```python
from build123d import *

# Parameters (mm, degrees)
F0_R     = 228.6
F3_DEPTH = 57.15
F4_DEPTH = 57.15


with BuildPart() as f2:
    # F2: sweep along a path in F1
    with BuildLine(Plane.XY) as f2_path:
        ThreePointArc((0, 457.2), (-323.2892203585, 323.2892203585), (-457.2, 0))
    # F0 (on Front) → F2 (sweep)
    with BuildSketch(Plane.XZ):
        with Locations((-685.8, 0)):
            Circle(F0_R)
    sweep(path=f2_path.line)

    # F3 (add): a face of the model
    f3_faces = [f2.faces().sort_by_distance(p)[0] for p in [
        (-685.8, 0, 0),
    ]]
    extrude(f3_faces, amount=F3_DEPTH)

    # F4 (add): a face of the model
    f4_faces = [f2.faces().sort_by_distance(p)[0] for p in [
        (0, 685.8, 0),
    ]]
    extrude(f4_faces, amount=F4_DEPTH)


solid = f2.part
```
Can you work these out from the model? Positions are in its coordinate system, mm. A direction names the side the tool comes from. Round coordinates to 2 decimals unless told otherwise and drop trailing zeros. Loops run counter-clockwise (first coordinate to the right, second up) from the corner with the lowest first, then second, coordinate; pieces in that order, holes last. Notation, with made-up numbers: (-27, 11) -> (18, 11) arc R23 cw to (18, 31) -> close; hole circle Ø3 at (-2, -27). An arc over 180 degrees is marked (long way). One line per item, written item: value. Start each with the question number.
1. If we section it at A-A, the plane z = 0: Write out the boundary of the cut face in (x, y), then the cut area to 3 significant figures.
2. If we section it at B-B, the plane z = -73: Write out the boundary of the cut face in (x, y).
3. If I drill on probe 1 along Y at (x, z) = (-88.5, -179); probe 2 along X at (y, z) = (804, -131); probe 3 along Y at (x, z) = (-276, -75), over which ranges is the centre line in solid material (lowest first)?
4. For faces 1 (the cylindrical face through (-854.288, -28.175, -154.499)), 2 (the flat face through (57.15, 689, 3)), 3 (the cylindrical face through (28.17, 562.91, -192.76)), which set-ups out of +Z, -Z, +X, -X, +Y, -Y let a thin tool reach every point of the face, with its end or its side?
5. For pin 1 (6 mm diameter, centred on x = -130, y = 644, fed in from -Z); pin 2 (1.5 mm diameter, centred on x = -151.5, y = 459.5, fed in from -Z); pin 3 (8 mm diameter, centred on x = -394, y = 596.5, fed in from +Z), each with a flat end and sliding along its axis, tell me the tip position at first contact or that it passes through.
Calculated:
1. outline: (-914.4, -57.15) -> (-457.2, -57.15) -> (-457.2, 0) arc R457.2 cw to (0, 457.2) -> (57.15, 457.2) -> (57.15, 914.4) -> (0, 914.4) arc R914.4 ccw to (-914.4, 0) -> close
1. area: 545,000 mm²
2. outline: (-902.43, -57.15) -> (-469.17, -57.15) -> (-469.17, 0) arc R469.17 cw to (0, 469.17) -> (57.15, 469.17) -> (57.15, 902.43) -> (0, 902.43) arc R902.43 ccw to (-902.43, 0) -> close
3. probe 1: y = 536.36 to 823.24
3. probe 2: x = -340.53 to 57.15
3. probe 3: y = 380.24 to 858.47
4. face 1: -Y
4. face 2: +Z, -Z, +X, +Y, -Y
4. face 3: +X
5. pin 1: stops at z = -227.14
5. pin 2: stops at z = -108.48
5. pin 3: stops at z = 227.22
